from build123d import *

# Parameters (mm, degrees)
SKETCH_2_R          = 6.5
SKETCH_2_R_2        = 1.3
SKETCH_2_R_3        = 2.5
EXTRUDE_1_DEPTH     = 7.5
SKETCH_10_R         = 1.3
CUT_EXTRUDE_2_DEPTH = 7.5
SKETCH_4_R          = 1.3
CUT_EXTRUDE_4_DEPTH = 7.5
CHAMFER_2_SIZE      = 0.2
CHAMFER_3_SIZE      = 0.2
CHAMFER_4_SIZE      = 0.5


with BuildPart() as part:
    # 草圖2 → 填料-伸長1 (new body)
    with BuildSketch(Plane.XY):
        with BuildLine():
            Line((40, 40), (5, 40))
            ThreePointArc((5, 40), (3.456243754, 39.57231737), (2.352645995, 38.411211101))
            Line((2.352645995, 38.411211101), (-24.912624764, -12.736929445))
            ThreePointArc((-24.912624764, -12.736929445), (-22.327787039, -24.202446867), (-10.606601718, -23.334523779))
            Line((-10.606601718, -23.334523779), (36.727922061, 24))
            Line((36.727922061, 24), (63.272077939, 24))
            Line((63.272077939, 24), (110.606601718, -23.334523779))
            ThreePointArc((110.606601718, -23.334523779), (122.823351862, -23.807584), (124.239699521, -11.663996007))
            Line((124.239699521, -11.663996007), (87.423045591, 38.768855581))
            ThreePointArc((87.423045591, 38.768855581), (86.358939524, 39.674562276), (85, 40))
            Line((85, 40), (40, 40))
        make_face()
        Circle(SKETCH_2_R, mode=Mode.SUBTRACT)
        with Locations((100, 0)):
            Circle(SKETCH_2_R, mode=Mode.SUBTRACT)
        with Locations((25, 35)):
            Circle(SKETCH_2_R_2, mode=Mode.SUBTRACT)
        with Locations((70, 35)):
            Circle(SKETCH_2_R_2, mode=Mode.SUBTRACT)
        with Locations((40, 35)):
            Circle(SKETCH_2_R_2, mode=Mode.SUBTRACT)
        with Locations((55, 35)):
            Circle(SKETCH_2_R_2, mode=Mode.SUBTRACT)
        with Locations((10, 35)):
            Circle(SKETCH_2_R_2, mode=Mode.SUBTRACT)
        with Locations((16.970562748, 16.970562748)):
            Circle(SKETCH_2_R_3, mode=Mode.SUBTRACT)
        with Locations((83.029437252, 16.970562748)):
            Circle(SKETCH_2_R_3, mode=Mode.SUBTRACT)
        with Locations((-16.970562748, -16.970562748)):
            Circle(SKETCH_2_R_3, mode=Mode.SUBTRACT)
        with Locations((116.970562748, -16.970562748)):
            Circle(SKETCH_2_R_3, mode=Mode.SUBTRACT)
    extrude(amount=EXTRUDE_1_DEPTH)

    # 草圖10 → 除料-伸長2 (cut)
    with BuildSketch(Plane(origin=(43.636038969, 43.636038969, 0), x_dir=(-0.70710678118655, 0.7071067811865451, 0), z_dir=(-0.7071067811865451, -0.70710678118655, 0))):
        with Locations(Location((-45.710678119, -3.75, 0), (0, 0, 180))):
            Circle(SKETCH_10_R)
        with Locations(Location((-35.710678119, -3.75, 0), (0, 0, 180))):
            Circle(SKETCH_10_R)
    extrude(amount=-CUT_EXTRUDE_2_DEPTH, mode=Mode.SUBTRACT)

    # 草圖4 → 除料-伸長4 (cut)
    with BuildSketch(Plane(origin=(6.363961031, -6.363961031, 0), x_dir=(-0.7071067811865464, -0.7071067811865488, 0), z_dir=(0.7071067811865488, -0.7071067811865464, 0))):
        with Locations(Location((-25, -3.75, 0), (0, 0, 180))):
            Circle(SKETCH_4_R)
        with Locations(Location((-35, -3.75, 0), (0, 0, 180))):
            Circle(SKETCH_4_R)
    extrude(amount=-CUT_EXTRUDE_4_DEPTH, mode=Mode.SUBTRACT)

    # 導角2
    chamfer_2_edges = [part.edges().sort_by_distance(p)[0] for p in [
        (67.968062812, 19.304015126, 3.75),
        (75.039130624, 12.232947315, 3.75),
    ]]
    chamfer(chamfer_2_edges, length=CHAMFER_2_SIZE)

    # 導角3
    chamfer_3_edges = [part.edges().sort_by_distance(p)[0] for p in [
        (23.122391745, 10.394469683, 3.75),
        (30.193459557, 17.465537495, 3.75),
    ]]
    chamfer(chamfer_3_edges, length=CHAMFER_3_SIZE)

    # 導角4
    chamfer_4_edges = [part.edges().sort_by_distance(p)[0] for p in [
        (14.470562748, 16.970562748, 0),
        (80.529437252, 16.970562748, 0),
        (114.470562748, -16.970562748, 0),
        (-19.470562748, -16.970562748, 0),
    ]]
    chamfer(chamfer_4_edges, length=CHAMFER_4_SIZE)


solid = part.part
Build history of the part. All positions in model axes, mm. A direction names the side the tool comes from. Give positions to 0.01 mm unless a question says otherwise; leave off trailing zeros. Order: outer loops, then holes, each group sorted by start corner. A loop starts at its lowest first (then second) coordinate and runs counter-clockwise, first axis right, second up. Notation, with made-up numbers: M 45,-1 L 96,-1 A11 cw 96,16 Z; hole C 62,34 d9. An arc over 180 degrees is marked long. Use one line per item in the form item = value.
Q1. Slice it at A-A, the plane y = 0. Write the cut outline in (x, z), and give its area (3 significant figures).
Conclusion:
outline = M -18.12,0 L -6.5,0 L -6.5,7.5 L -18.12,7.5 Z; M 6.5,0 L 12.73,0 L 12.73,7.5 L 6.5,7.5 Z; M 87.27,0 L 93.5,0 L 93.5,7.5 L 87.27,7.5 Z; M 106.5,0 L 115.72,0 L 115.72,7.5 L 106.5,7.5 Z
area = 250 mm2
Q2. Wall check: probe 1 along X at (y, z) = (-6, 3); probe 2 along X at (y, z) = (-4, 6); probe 3 along Y at (x, z) = (47, 7). Give the ranges that are in metal, low to high.
Conclusion:
probe_1 = -21.32 to -2.5, 2.5 to 6.73, 93.27 to 97.5, 102.5 to 120.1
probe_2 = -20.26 to -5.12, 5.12 to 8.73, 91.27 to 94.88, 105.12 to 118.64
probe_3 = 24 to 40
Q3. Slice it at B-B, the plane y = 30.5. Write the cut outline in (x, z).
Conclusion:
outline = M -1.86,0 L 93.46,0 L 93.46,7.5 L -1.86,7.5 Z
Q4. Pin check, flat tips, straight feed: P1, Ø1, axis at x = 42.5, z = 5.5, coming from the -Y side; P2, Ø8, axis at x = 100, y = 0, coming from the +Z side (3 decimals); P3, Ø1, axis at y = 13, z = 4.5, coming from the +X side. Stop position of each tip, or through.
Conclusion:
P1 = 24
P2 = through
P3 = 106.6
Q5. Which spindle directions (+Z, -Z, +X, -X, +Y, -Y) get a long thin tool onto all of the face, cutting with end or side? Do faces 4 (the cylindrical face through (3.5, 39.6, 3.7)), 5 (the flat face through (50, 24, 4)). Say none if no direction does.
Conclusion:
face_4 = +Z, -Z, -X, +Y
face_5 = +Z, -Z, -Y
Q6. Pull direction X, two halves, no side cores. Call faces 1 (the flat face through (44, 24.3, 0)), 2 (the flat face through (12.73, 0, 3.7)), 3 (the flat face through (-11.089, 13.195, 3.698)): released by +X, released by -X, zero draft, split by the parting line, or undercut.
Conclusion:
face_1 = zero draft
face_2 = undercut
face_3 = released by -X
